Read the model definition and answer for the solid it produces. Units are mm, in the model's axes. Give positions to 0.01 mm unless a question says otherwise; leave off trailing zeros. Write each loop counter-clockwise with the first axis right and the second up, starting at its lowest first coordinate (ties: lowest second). Pieces come first, ordered by that corner, then holes. Notation, with made-up numbers: M 73.25,37 L 117.25,37 A33 ccw 117.25,65 Z; hole C -27.5,-12.75 d2. An arc over 180 degrees is marked long. Use a Markdown table: item, result. Add a question column.
Item 1: A cutting plane is placed at B-B on x = 0. Determine the outline of the cut face in (y, z).
Item 2: A cutting plane is placed at C-C on y = 15. Determine the outline of the cut face in (x, z).
Item 3: Given P1, Ø1.5, axis at y = 26.5, z = 15, coming from the +X side; P2, Ø10, axis at x = -5.5, z = 5, coming from the +Y side, each flat-ended and moving along its own axis, determine where each tip first touches the part or whether it passes through.
Item 4: A cutting plane is placed at A-A on z = 0. Determine the outline of the cut face in (x, y).
Item 5: A cutting plane is placed at D-D on z = 18. Determine the outline of the cut face in (x, y).
Item 6: Consider probe 1 along Z at (x, y) = (2, 12); probe 2 along X at (y, z) = (10, -3.5); probe 3 along X at (y, z) = (22, 8.5). Determine where each line is inside the solid, lowest interval first. Write a range as [from, to].
Item 7: The mould has two halves that part along Z. Classify faces 1 (the cylindrical face through (14.648, 15.97, -20.775)), 2 (the cylindrical face through (20.775, 15.97, 14.648)), 3 (the cylindrical face through (14.579, 15.53, -16.345)): pulls with the +Z half, pulls with the -Z half, needs draft (parallel to the pull), parting line crosses it, or undercut.
from build123d import *

# Parameters (mm, degrees)
SKETCH_1_R      = 1.25
SKETCH_1_R_2    = 15.5
EXTRUDE_1_DEPTH = 31.5
FILLET_1_R      = 4


with BuildPart() as part:
    # Эскиз1 → Бобышка-Вытянуть1 (new body)
    with BuildSketch(Plane(origin=(0, 0, 0), x_dir=(1, 0, 0), z_dir=(0, 1, 0))):
        with BuildLine():
            Line((-14.641038215, -21), (14.641038215, -21))
            ThreePointArc((14.641038215, -21), (18.101933598, -18.101933598), (21, -14.641038215))
            Line((21, -14.641038215), (21, 14.641038215))
            ThreePointArc((21, 14.641038215), (18.101933598, 18.101933598), (14.641038215, 21))
            Line((14.641038215, 21), (-14.641038215, 21))
            ThreePointArc((-14.641038215, 21), (-18.101933598, 18.101933598), (-21, 14.641038215))
            Line((-21, 14.641038215), (-21, -14.641038215))
            ThreePointArc((-21, -14.641038215), (-18.101933598, -18.101933598), (-14.641038215, -21))
        make_face()
        with Locations((-15.5, 15.5)):
            Circle(SKETCH_1_R, mode=Mode.SUBTRACT)
        with Locations((15.5, 15.5)):
            Circle(SKETCH_1_R, mode=Mode.SUBTRACT)
        with Locations((15.5, -15.5)):
            Circle(SKETCH_1_R, mode=Mode.SUBTRACT)
        with Locations((-15.5, -15.5)):
            Circle(SKETCH_1_R, mode=Mode.SUBTRACT)
        Circle(SKETCH_1_R_2, mode=Mode.SUBTRACT)
    extrude(amount=EXTRUDE_1_DEPTH)

    # Скругление1
    fillet_1_edges = [part.edges().sort_by_distance(p)[0] for p in [
        (21, 15.75, -14.641038215),
        (21, 15.75, 14.641038215),
        (14.641038215, 15.75, 21),
        (-14.641038215, 15.75, 21),
        (-21, 15.75, 14.641038215),
        (-21, 15.75, -14.641038215),
        (-14.641038215, 15.75, -21),
        (14.641038215, 15.75, -21),
    ]]
    fillet(fillet_1_edges, radius=FILLET_1_R)


solid = part.part
Filled in:
| question | item | result |
|---|---|---|
| 1 | outline | M 0,-21 L 31.5,-21 L 31.5,-15.5 L 0,-15.5 Z; M 0,15.5 L 31.5,15.5 L 31.5,21 L 0,21 Z |
| 2 | outline | M -21,-13.33 A4 ccw -20.15,-15.79 A25.6 ccw -15.79,-20.15 A4 ccw -13.33,-21 L 13.33,-21 A4 ccw 15.79,-20.15 A25.6 ccw 20.15,-15.79 A4 ccw 21,-13.33 L 21,13.33 A4 ccw 20.15,15.79 A25.6 ccw 15.79,20.15 A4 ccw 13.33,21 L -13.33,21 A4 ccw -15.79,20.15 A25.6 ccw -20.15,15.79 A4 ccw -21,13.33 Z; hole C -15.5,-15.5 d2.5; hole C -15.5,15.5 d2.5; hole C 0,0 d31; hole C 15.5,-15.5 d2.5; hole C 15.5,15.5 d2.5 |
| 3 | P1 | x = 20.89 |
| 3 | P2 | through |
| 4 | outline | M -21,0 L -15.5,0 L -15.5,31.5 L -21,31.5 Z; M 15.5,0 L 21,0 L 21,31.5 L 15.5,31.5 Z |
| 5 | outline | M -18.2,0 L 18.2,0 L 18.2,31.5 L -18.2,31.5 Z |
| 6 | probe 1 | [-21, -15.37], [15.37, 21] |
| 6 | probe 2 | [-21, -15.1], [15.1, 21] |
| 6 | probe 3 | [-21, -12.96], [12.96, 21] |
| 7 | face 1 | pulls with the -Z half |
| 7 | face 2 | pulls with the +Z half |
| 7 | face 3 | undercut |
